Part model, mm, in its own coordinate system. Round coordinates to 2 decimals unless told otherwise and drop trailing zeros. Loops run counter-clockwise (first coordinate to the right, second up) from the corner with the lowest first, then second, coordinate; pieces in that order, holes last. Notation, with made-up numbers: (-14, 13.25) - (6, 13.25) arc R20 cw to (6, 17.25) - close; hole circle Ø9 at (81.5, 50). An arc over 180 degrees is marked (long way). Put each result on its own line as item: value.
from build123d import *

# Parameters (mm, degrees)
F0_W     = 360
F0_H     = 0.278708
F0_H_2   = 399.721292
F0_W_2   = 60
F0_H_3   = 120
F0_W_3   = 40
F0_H_4   = 40
F0_H_5   = 39.721292
F1_DEPTH = 6
F2_D     = 160


with BuildPart() as f1:
    # F0 (on Top) → F1 (new body)
    with BuildSketch(Plane.XY):
        with Locations((0, -199.860646)):
            Rectangle(F0_W, F0_H)
        with Locations((0, 0.139354)):
            Rectangle(F0_W, F0_H_2)
        with Locations((-130, -120)):
            Rectangle(F0_W_2, F0_H_3, mode=Mode.SUBTRACT)
        with Locations((130, -120)):
            Rectangle(F0_W_2, F0_H_3, mode=Mode.SUBTRACT)
        with Locations((-130, 120)):
            Rectangle(F0_W_2, F0_H_3, mode=Mode.SUBTRACT)
        with Locations((130, 120)):
            Rectangle(F0_W_2, F0_H_3, mode=Mode.SUBTRACT)
        with Locations((-200, 0.139354)):
            Rectangle(F0_W_3, F0_H_2)
        with Locations((0, 220)):
            Rectangle(F0_W, F0_H_4)
        with Locations((0, -219.860646)):
            Rectangle(F0_W, F0_H_5)
        with Locations((200, 0.139354)):
            Rectangle(F0_W_3, F0_H_2)
    extrude(amount=F1_DEPTH)

    # F2 (through all)
    with Locations(Plane(origin=(0, 0, 0), x_dir=(1, 0, 0), z_dir=(0, 0, -1))):
        with Locations((0, 0)):
            Hole(F2_D / 2)


solid = f1.part
1. Probe line 1 along X through (y, z) = (-126.5, 2.95); line 2 along Y through (x, z) = (116, 4.6); line 3 along Y through (x, z) = (0, 1.8). List the from-to ranges inside material, lowest first. Write a range as [from, to].
A:
line 1: x = [-220, -160], [-100, 100], [160, 220]
line 2: y = [-239.72, -180], [-60, 60], [180, 240]
line 3: y = [-239.72, -80], [80, 240]
2. Band-saw the part on B-B (x = 0). List the corners of the cut face in (y, z).
A:
outline: (-239.72, 0) - (-80, 0) - (-80, 6) - (-239.72, 6) - close; (80, 0) - (240, 0) - (240, 6) - (80, 6) - close
3. Band-saw the part on C-C (y = 0). List the corners of the cut face in (x, z).
A:
outline: (-220, 0) - (-80, 0) - (-80, 6) - (-220, 6) - close; (80, 0) - (220, 0) - (220, 6) - (80, 6) - close
4. Band-saw the part on A-A (x = 129). List the corners of the cut face in (y, z).
A:
outline: (-239.72, 0) - (-180, 0) - (-180, 6) - (-239.72, 6) - close; (-60, 0) - (60, 0) - (60, 6) - (-60, 6) - close; (180, 0) - (240, 0) - (240, 6) - (180, 6) - close
5. Band-saw the part on D-D (z = 3.5). Give the number of separate pieces and of enclosed holes in the cut face, plus the area to 3 significant figures.
A:
separate pieces: 1
enclosed holes: 5
area: 156,000 mm²
6. Pin check, flat tips, straight feed: P1, Ø4, axis at x = -61.5, y = 46, coming from the -Z side; P2, Ø3, axis at y = -217.5, z = 3, coming from the -X side; P3, Ø1.8, axis at y = -229.5, z = 2.5, coming from the +X side. Stop position of each tip, or through.
A:
P1: passes through
P2: stops at x = -180
P3: stops at x = 180
7. Two-plate mould, pull along X, no slides. Class faces 1 (the flat face through (95, 3, 0)), 2 (the cylindrical face through (17.34, 78.1, 3.04)): pulls with the +X half, pulls with the -X half, needs draft (parallel to the pull), parting line crosses it, or undercut.
A:
face 1: needs draft
face 2: undercut
